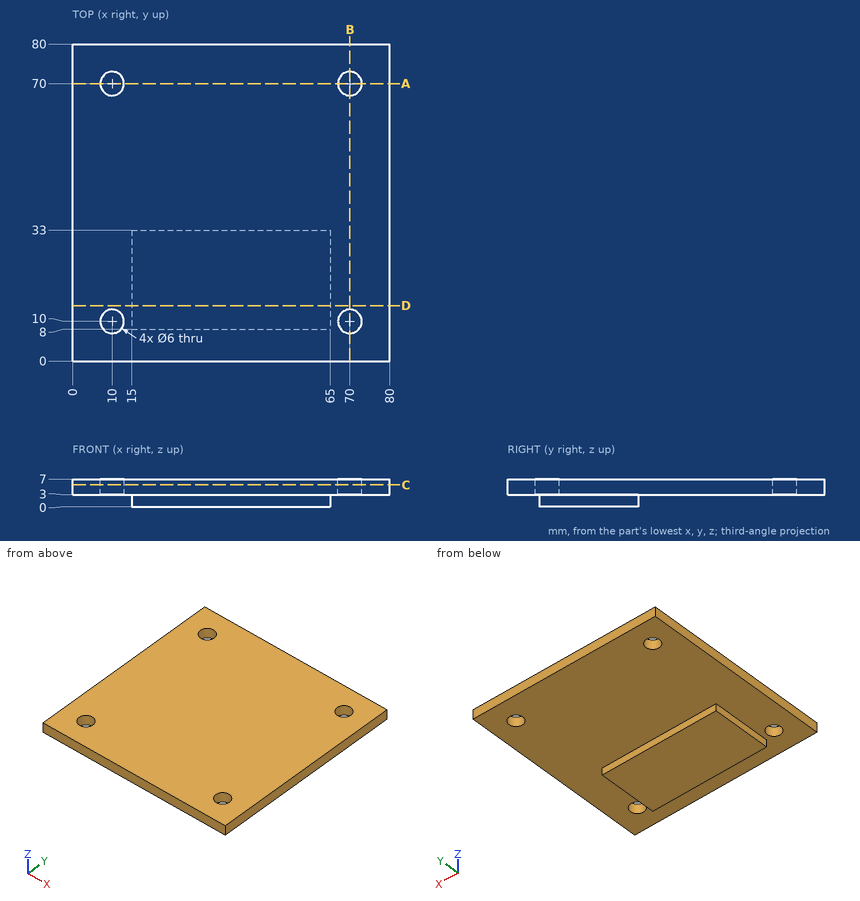
Geometry: see drawing. Coordinates: mm, zero at the bounding-box minimum. Give positions to 0.01 mm unless a question says otherwise; leave off trailing zeros. Order: outer loops, then holes, each group sorted by start corner. A loop starts at its lowest first (then second) coordinate and runs counter-clockwise, first axis right, second up. Notation, with made-up numbers: (-13, -22) -> (24, -22) arc R21 ccw to (24, -10) -> close; hole circle Ø11 at (39.5, 47.25). An arc over 180 degrees is marked (long way). Write each question's results on one line, items separated by ' | '. Start each with the question number.
1) Section D-D (y = 14). Return loops of the section in (x, z), then the cut area to 3 significant figures.
2) Line query: line 1 (X direction, y = 70, z = 4); line 2 (Y direction, x = 9, z = 5.75). Output: solid intervals per line, ascending. Write a range as from..to.
3) First-contact query: pin 1 (1.5 mm diameter, centred on y = 15, z = 1, fed in from +X); pin 2 (7 mm diameter, centred on x = 10, y = 70, fed in from -Z); pin 3 (0.9 mm diameter, centred on y = 23.5, z = 1, fed in from -X); pin 4 (2.5 mm diameter, centred on x = 29.5, z = 2, fed in from -Y). Flat tips, straight axial feed; report the tip coordinate or a pass-through.
4) Section A-A (y = 70). Return loops of the section in (x, z).
5) Section C-C (z = 5.5). Return loops of the section in (x, y).
Calculated:
1) outline: (0, 3) -> (15, 3) -> (15, 0) -> (65, 0) -> (65, 3) -> (80, 3) -> (80, 7) -> (0, 7) -> close | area: 470 mm2
2) line 1: 0..7, 13..67, 73..80 | line 2: 0..7.17, 12.83..67.17, 72.83..80
3) pin 1: x = 65 | pin 2: z = 3 | pin 3: x = 15 | pin 4: y = 0
4) outline: (0, 3) -> (7, 3) -> (7, 7) -> (0, 7) -> close; (13, 3) -> (67, 3) -> (67, 7) -> (13, 7) -> close; (73, 3) -> (80, 3) -> (80, 7) -> (73, 7) -> close
5) outline: (0, 0) -> (80, 0) -> (80, 80) -> (0, 80) -> close; hole circle Ø6 at (10, 10); hole circle Ø6 at (10, 70); hole circle Ø6 at (70, 10); hole circle Ø6 at (70, 70)
